Design review of the part built by this model. Coordinates are the model's own, in mm. Give positions to 0.01 mm unless a question says otherwise; leave off trailing zeros. Loops run counter-clockwise (first coordinate to the right, second up) from the corner with the lowest first, then second, coordinate; pieces in that order, holes last. Notation, with made-up numbers: (-22, 84.25) -> (19, 84.25) arc R24 cw to (19, 118.25) -> close; hole circle Ø1 at (-27, 38). An arc over 180 degrees is marked (long way). Use CSV: the item, a comma, the result in double quotes. Start each with the question number.
Item 1: We need section A-A (y = 0.9). State the section outline as (x, z) points.
Item 2: Clearance check with flat-ended pins moving along their axes: pin 1 (12 mm diameter, centred on x = -21.5, z = 25.5, fed in from -Y); pin 2 (0.5 mm diameter, centred on y = 0.5, z = 2, fed in from -X). State where each tip first meets the part, or that it passes through.
Item 3: Wall thickness on line 1 along Z through (x, y) = (-7, 0.4); line 2 along Z through (x, y) = (21, 1.1); line 3 along X through (y, z) = (1.15, 7.5): over which ranges is each line inside the solid? List them lowest first. Write a range as from..to.
Item 4: We need section C-C (x = 23.5). State the section outline as (y, z) points.
Item 5: We need section B-B (z = 4.5). State the section outline as (x, y) points, plus the area to 3 significant figures.
from build123d import *

# Parameters (mm, degrees)
BOSS_EXTRUDE1_DEPTH = 1.5


with BuildPart() as part:
    # Sketch1 → Boss-Extrude1 (new body)
    with BuildSketch(Plane(origin=(0, 0, 0), x_dir=(1, 0, 0), z_dir=(0, 1, 0))):
        with BuildLine():
            Line((29.399956383, -10.909440226), (29.399956383, -35.694042527))
            Line((29.399956383, -35.694042527), (-29.399956383, -35.694042527))
            Line((-29.399956383, -35.694042527), (-29.399956383, -10.909440226))
            ThreePointArc((-29.399956383, -10.909440226), (-29.130344067, -9.933819399), (-28.398023754, -9.235082141))
            ThreePointArc((-28.398023754, -9.235082141), (-18.42847588, -4.996086333), (-7.859761529, -2.616328524))
            ThreePointArc((-7.859761529, -2.616328524), (-7.735749713, -2.604086526), (-7.611202142, -2.6))
            Line((-7.611202142, -2.6), (-6.8, -2.6))
            Line((-6.8, -2.6), (-6.8, -1.6))
            Line((-6.8, -1.6), (6.8, -1.6))
            Line((6.8, -1.6), (6.8, -2.6))
            Line((6.8, -2.6), (7.611202142, -2.6))
            ThreePointArc((7.611202142, -2.6), (7.735749713, -2.604086526), (7.859761529, -2.616328524))
            ThreePointArc((7.859761529, -2.616328524), (18.42847588, -4.996086333), (28.398023754, -9.235082141))
            ThreePointArc((28.398023754, -9.235082141), (29.130344067, -9.933819399), (29.399956383, -10.909440226))
        make_face()
    extrude(amount=BOSS_EXTRUDE1_DEPTH)


solid = part.part
Results found:
1,outline,"(-29.4, 10.91) arc R1.9 ccw to (-28.4, 9.24) arc R60.08 ccw to (-7.86, 2.62) arc R1.9 ccw to (-7.61, 2.6) -> (-6.8, 2.6) -> (-6.8, 1.6) -> (6.8, 1.6) -> (6.8, 2.6) -> (7.61, 2.6) arc R1.9 ccw to (7.86, 2.62) arc R60.08 ccw to (28.4, 9.24) arc R1.9 ccw to (29.4, 10.91) -> (29.4, 35.69) -> (-29.4, 35.69) -> close"
2,pin 1,"y = 0"
2,pin 2,"x = -6.8"
3,line 1,"2.6..35.69"
3,line 2,"5.89..35.69"
3,line 3,"-24.89..24.89"
4,outline,"(0, 6.89) -> (1.5, 6.89) -> (1.5, 35.69) -> (0, 35.69) -> close"
5,outline,"(-16.81, 0) -> (16.81, 0) -> (16.81, 1.5) -> (-16.81, 1.5) -> close"
5,area,"50.4 mm²"
